The listing builds one solid part. Answer for the finished solid, in the listing's coordinates (mm). Face numbers are marked on the shaded views. A direction names the side the tool comes from. Round coordinates to 2 decimals unless told otherwise and drop trailing zeros. Loops run counter-clockwise (first coordinate to the right, second up) from the corner with the lowest first, then second, coordinate; pieces in that order, holes last. Notation, with made-up numbers: (27.25, 41) -> (67.25, 41) arc R25 cw to (67.25, 56) -> close; hole circle Ø2 at (55.5, 37). An arc over 180 degrees is marked (long way). Write each question's results on one line, items separated by ' | '. Start each with the question number.
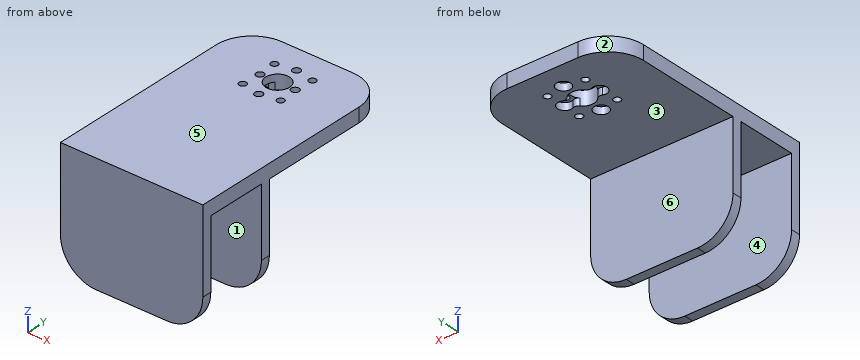
from build123d import *

# Parameters (mm, degrees)
SKETCH1_W           = 60
SKETCH1_H           = 60
SKETCH1_R           = 5
SKETCH1_R_2         = 1.65
SKETCH1_R_3         = 1.5
BOSS_EXTRUDE1_DEPTH = 6
SKETCH2_W           = 6
SKETCH2_H           = 25.5
BOSS_EXTRUDE2_DEPTH = 60
FILLET1_R           = 15
SKETCH3_R           = 3
CUT_EXTRUDE1_DEPTH  = 3
FILLET2_R           = 2


with BuildPart() as part:
    # Sketch1 → Boss-Extrude1 (new body)
    with BuildSketch(Plane.XY):
        with Locations((30, 30)):
            Rectangle(SKETCH1_W, SKETCH1_H)
        with Locations((30, 40)):
            Circle(SKETCH1_R, mode=Mode.SUBTRACT)
        with Locations((30, 49.5)):
            Circle(SKETCH1_R_2, mode=Mode.SUBTRACT)
        with Locations((30, 30.5)):
            Circle(SKETCH1_R_2, mode=Mode.SUBTRACT)
        with Locations((22.6, 40)):
            Circle(SKETCH1_R_2, mode=Mode.SUBTRACT)
        with Locations((37.4, 40)):
            Circle(SKETCH1_R_2, mode=Mode.SUBTRACT)
        with Locations((22, 48)):
            Circle(SKETCH1_R_3, mode=Mode.SUBTRACT)
        with Locations((38, 48)):
            Circle(SKETCH1_R_3, mode=Mode.SUBTRACT)
        with Locations((38, 32)):
            Circle(SKETCH1_R_3, mode=Mode.SUBTRACT)
        with Locations((22, 32)):
            Circle(SKETCH1_R_3, mode=Mode.SUBTRACT)
    extrude(amount=BOSS_EXTRUDE1_DEPTH)

    # Sketch2 → Boss-Extrude2 (add)
    with BuildSketch(Plane(origin=(60, 0, 0), x_dir=(0, 0, -1), z_dir=(1, 0, 0))):
        Polygon((44, 0), (-6, 0), (-6, -4), (0, -4), (44, -4), align=None)
        with Locations((-3, -16.75)):
            Rectangle(SKETCH2_W, SKETCH2_H)
        Polygon((0, -29.5), (-6, -29.5), (-6, -33.5), (44, -33.5), (44, -29.5), align=None)
    extrude(amount=-BOSS_EXTRUDE2_DEPTH)

    # Fillet1
    fillet1_edges = [part.edges().sort_by_distance(p)[0] for p in [
        (60, -2, -44),
        (0, -31.5, -44),
        (0, -2, -44),
        (60, -31.5, -44),
        (0, 60, 3),
        (60, 60, 3),
    ]]
    fillet(fillet1_edges, radius=FILLET1_R)

    # Sketch3 → Cut-Extrude1 (cut)
    with BuildSketch(Plane(origin=(0, 0, 0), x_dir=(-1, 0, 0), z_dir=(0, 0, -1))):
        with Locations((-30, 49.5)):
            Circle(SKETCH3_R)
        with Locations((-22.6, 40)):
            Circle(SKETCH3_R)
        with Locations((-30, 30.5)):
            Circle(SKETCH3_R)
        with Locations((-37.4, 40)):
            Circle(SKETCH3_R)
    extrude(amount=-CUT_EXTRUDE1_DEPTH, mode=Mode.SUBTRACT)

    # Fillet2
    fillet2_edges = [part.edges().sort_by_distance(p)[0] for p in [
        (34.781081081, 41.463305743, 1.5),
        (34.781081081, 38.536694257, 1.5),
        (25.218918919, 38.536694257, 1.5),
        (25.218918919, 41.463305743, 1.5),
    ]]
    fillet(fillet2_edges, radius=FILLET2_R)


solid = part.part
Item 1: The part is cut by section A-A, the plane y = 40. Give the vertices of the cut face in (x, z).
Item 2: Each of these flat-tipped pins is pushed along its axis until it touches: pin 1 Ø9.5 at (x, y) = (22.6, 40) entering from -Z; pin 2 Ø2.5 at (x, y) = (38, 32) entering from -Z; pin 3 Ø5 at (x, y) = (38, 48) entering from +Z; pin 4 Ø3 at (x, y) = (22, 40) entering from -Z. Where does it stop, or does it pass through?
Item 3: Determine the mould class of the marked faces 1, 2 and 3 for opening direction Y: +Y half, -Y half, draft (parallel to the pull), parting line (faces both ways), or undercut.
Item 4: The part is cut by section C-C, the plane x = 30. Give the number of separate pieces and of enclosed holes in the cut face, plus the area to 3 significant figures.
Item 5: For the marked faces 4, 5 and 6, determine the directions among +Z, -Z, +X, -X, +Y, -Y from which every point of the face is accessible in a straight line to the end or side of a thin tool.
Item 6: The part is cut by section D-D, the plane x = 22. Give the vertices of the cut face in (y, z), plus the area to 3 significant figures.
Item 7: Straight lines are drawn through the part: L1, parallel to X at y = 40, z = 4.3; L2, parallel to Y at x = 32.5, z = -22.5; L3, parallel to Y at x = 22, z = 1.9. For each, find the intervals that lie inside material, in ascending order. Write a range as [from, to].
Item 8: The part is cut by section B-B, the plane z = -16. Give the vertices of the cut face in (x, y), plus the area to 3 significant figures.
Report:
1) outline: (0, 0) -> (19.6, 0) -> (19.6, 3) -> (20.95, 3) -> (20.95, 6) -> (0, 6) -> close; (24.25, 3) -> (25, 3) -> (25, 6) -> (24.25, 6) -> close; (35, 3) -> (35.75, 3) -> (35.75, 6) -> (35, 6) -> close; (39.05, 3) -> (40.4, 3) -> (40.4, 0) -> (60, 0) -> (60, 6) -> (39.05, 6) -> close
2) pin 1: stops at z = 0 | pin 2: passes through | pin 3: stops at z = 6 | pin 4: stops at z = 3
3) face 1: undercut | face 2: +Y half | face 3: draft
4) separate pieces: 4 | enclosed holes: 0 | area: 797 mm2
5) face 4: -Z, +X, -X | face 5: +Z, +X, -X, +Y, -Y | face 6: -Z, +X, -X, +Y
6) outline: (-33.5, -44) -> (-29.5, -44) -> (-29.5, 0) -> (-4, 0) -> (-4, -44) -> (0, -44) -> (0, 0) -> (30.5, 0) -> (30.5, 6) -> (-33.5, 6) -> close; (33.5, 0) -> (37.06, 0) -> (37.06, 3) -> (38.46, 3) -> (38.46, 6) -> (33.5, 6) -> close; (41.54, 3) -> (42.94, 3) -> (42.94, 0) -> (46.5, 0) -> (46.5, 6) -> (41.54, 6) -> close; (49.5, 0) -> (60, 0) -> (60, 6) -> (49.5, 6) -> close | area: 850 mm2
7) L1: x = [0, 20.95], [24.25, 25], [35, 35.75], [39.05, 60] | L2: y = [-33.5, -29.5], [-4, 0] | L3: y = [-33.5, 30.5], [33.5, 37.06], [42.94, 46.5], [49.5, 60]
8) outline: (0, -33.5) -> (60, -33.5) -> (60, -29.5) -> (0, -29.5) -> close; (0, -4) -> (60, -4) -> (60, 0) -> (0, 0) -> close | area: 480 mm2
